Work out the finished part from the listing and answer in its coordinate system (mm). Face numbers are marked on the shaded views. Give positions to 0.01 mm unless a question says otherwise; leave off trailing zeros. Order: outer loops, then holes, each group sorted by start corner. A loop starts at its lowest first (then second) coordinate and runs counter-clockwise, first axis right, second up. Notation, with made-up numbers: M -26.75,-8.75 L 19.25,-8.75 A12 cw 19.25,1.25 Z; hole C 66.25,60.5 d6. An arc over 180 degrees is marked long. One line per item, written item: value.
from build123d import *

# Parameters (mm, degrees)
SKETCH_1_R      = 13
SKETCH_1_R_2    = 8.5
EXTRUDE_1_DEPTH = 5
EXTRUDE_START   = -1.1
SKETCH_2_R      = 14
SKETCH_2_R_2    = 13
EXTRUDE_2_DEPTH = 1.1
FILLET_1_R      = 0.3


with BuildPart() as part:
    # 草图1 → 凸台-拉伸1 (new body)
    with BuildSketch(Plane.XY):
        Circle(SKETCH_1_R)
        Circle(SKETCH_1_R_2, mode=Mode.SUBTRACT)
    extrude(amount=EXTRUDE_1_DEPTH)

    # 草图2 → 凸台-拉伸2 (add)
    with BuildSketch(Plane.XY.offset(5).offset(EXTRUDE_START)):
        Circle(SKETCH_2_R)
        Circle(SKETCH_2_R_2, mode=Mode.SUBTRACT)
    extrude(amount=EXTRUDE_2_DEPTH)

    # 圆角1
    fillet_1_edges = [part.edges().sort_by_distance(p)[0] for p in [
        (-13, 0, 0),
    ]]
    fillet(fillet_1_edges, radius=FILLET_1_R)


solid = part.part
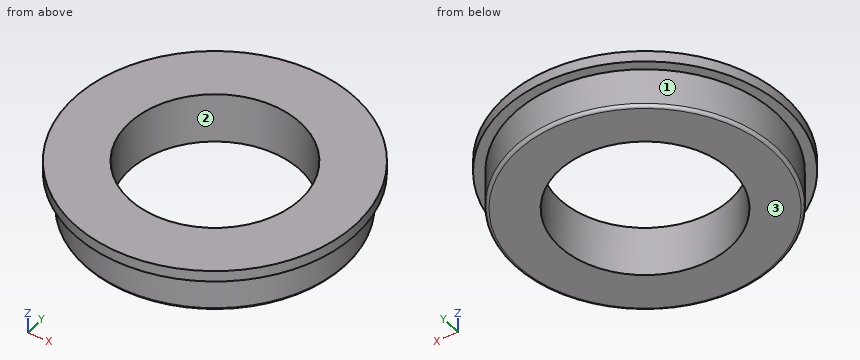
(1) Section C-C, the plane z = 2.9 is taken. Give the vertices of the cut face in (x, y).
Findings:
outline: C 0,0 d26; hole C 0,0 d17
(2) Find the intervals of material crossed by probe 1 along Y at (x, z) = (0, 3.2); probe 2 along X at (y, z) = (4, 4.6); probe 3 along Y at (x, z) = (7, 2.6), in increasing order. Write a range as from..to.
Findings:
probe 1: y = -13..-8.5, 8.5..13
probe 2: x = -13.42..-7.5, 7.5..13.42
probe 3: y = -10.95..-4.82, 4.82..10.95
(3) Determine the mould class of the marked faces 1, 2 and 3 for opening direction Y: pulls with the +Y half, pulls with the -Y half, needs draft (parallel to the pull), parting line crosses it, or undercut.
Findings:
face 1: parting line crosses it
face 2: undercut
face 3: needs draft
(4) Given P1, Ø3, axis at y = -3, z = 0.5, coming from the +X side; P2, Ø1, axis at y = 7, z = 1.5, coming from the -X side, each flat-ended and moving along its own axis, determine where each tip first touches the part or whether it passes through.
Findings:
P1: stops at x = 12.91
P2: stops at x = -11.26
(5) Section D-D, the plane z = 4.5 is taken. Give the vertices of the cut face in (x, y).
Findings:
outline: C 0,0 d28; hole C 0,0 d17
(6) Section A-A, the plane x = 0 is taken. Give the vertices of the cut face in (y, z), then the cut area to 3 significant figures.
Findings:
outline: M -14,3.9 L -13,3.9 L -13,0.3 A0.3 ccw -12.7,0 L -8.5,0 L -8.5,5 L -14,5 Z; M 8.5,0 L 12.7,0 A0.3 ccw 13,0.3 L 13,3.9 L 14,3.9 L 14,5 L 8.5,5 Z
area: 47.2 mm^2
